Geometry check sheet. Reference: the model listing, model coordinates, mm. Face numbers are marked on the shaded views. A direction names the side the tool comes from. Give positions to 0.01 mm unless a question says otherwise; leave off trailing zeros. Write each loop counter-clockwise with the first axis right and the second up, starting at its lowest first coordinate (ties: lowest second). Pieces come first, ordered by that corner, then holes. Notation, with made-up numbers: (38.25, -8.5) - (68.25, -8.5) arc R14 cw to (68.25, 11.5) - close; hole circle Ø3 at (-16, 7.25). An arc over 180 degrees is marked (long way). Use a Markdown table: item, result.
```python
from build123d import *

# Parameters (mm, degrees)
SKETCH1_R           = 1.5
BOSS_EXTRUDE1_DEPTH = 3


with BuildPart() as part:
    # Sketch1 → Boss-Extrude1 (new body)
    with BuildSketch(Plane.XY):
        with BuildLine():
            Line((84.808392572, 18.957643404), (78, 19.433732591))
            Line((78, 19.433732591), (78, 13))
            ThreePointArc((78, 13), (81.889087297, 11.389087297), (83.5, 7.5))
            Line((83.5, 7.5), (83.5, -7.5))
            ThreePointArc((83.5, -7.5), (81.889087297, -11.389087297), (78, -13))
            Line((78, -13), (78, -19.433732591))
            Line((78, -19.433732591), (84.808392572, -18.957643404))
            ThreePointArc((84.808392572, -18.957643404), (87.805263235, -17.68554728), (89.383648968, -14.838064041))
            Line((89.383648968, -14.838064041), (91.846905706, -0.868240888))
            ThreePointArc((91.846905706, -0.868240888), (91.922866941, 0), (91.846905706, 0.868240888))
            Line((91.846905706, 0.868240888), (89.383648968, 14.838064041))
            ThreePointArc((89.383648968, 14.838064041), (87.805263235, 17.68554728), (84.808392572, 18.957643404))
        make_face()
        with Locations((81, -16)):
            Circle(SKETCH1_R, mode=Mode.SUBTRACT)
        with Locations((81, 16)):
            Circle(SKETCH1_R, mode=Mode.SUBTRACT)
    extrude(amount=BOSS_EXTRUDE1_DEPTH)


solid = part.part
```
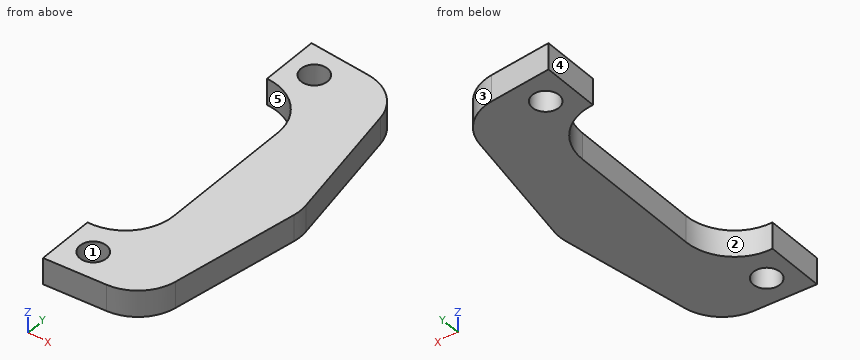
1) Section check B-B on x = 81. Record the boundary of the cut face in (y, z), then the cut area to 3 significant figures.
Working result:
| item | result |
|---|---|
| outline | (-19.22, 0) - (-17.5, 0) - (-17.5, 3) - (-19.22, 3) - close; (-14.5, 0) - (-12.11, 0) - (-12.11, 3) - (-14.5, 3) - close; (12.11, 0) - (14.5, 0) - (14.5, 3) - (12.11, 3) - close; (17.5, 0) - (19.22, 0) - (19.22, 3) - (17.5, 3) - close |
| area | 24.7 mm² |
2) Set-up check for the marked faces 1 and 2: record each of +Z, -Z, +X, -X, +Y, -Y from which the full face is reachable in a straight line by a thin tool's end or side.
Working result:
| item | result |
|---|---|
| face 1 | +Z, -Z |
| face 2 | +Z, -Z, -X |
3) Section check C-C on y = 16. Record the boundary of the cut face in (x, z), then the cut area to 3 significant figures.
Working result:
| item | result |
|---|---|
| outline | (78, 0) - (79.5, 0) - (79.5, 3) - (78, 3) - close; (82.5, 0) - (89.03, 0) - (89.03, 3) - (82.5, 3) - close |
| area | 24.1 mm² |
4) Section check A-A on z = 0.6. Record the boundary of the cut face in (x, y).
Working result:
| item | result |
|---|---|
| outline | (78, -19.43) - (84.81, -18.96) arc R5 ccw to (89.38, -14.84) - (91.85, -0.87) arc R5 ccw to (91.85, 0.87) - (89.38, 14.84) arc R5 ccw to (84.81, 18.96) - (78, 19.43) - (78, 13) arc R5.5 cw to (83.5, 7.5) - (83.5, -7.5) arc R5.5 cw to (78, -13) - close; hole circle Ø3 at (81, -16); hole circle Ø3 at (81, 16) |
5) Depth check by flat-ended pin: P1, Ø3.5, axis at x = 81, y = -16, coming from the +Z side; P2, Ø1.5, axis at y = -3, z = 1, coming from the -X side. Enter the tip coordinate at first touch or a pass-through.
Working result:
| item | result |
|---|---|
| P1 | stops at z = 3 |
| P2 | stops at x = 83.5 |
6) Mould release check, pull along Y, two halves, no side actions. Record for the marked faces 3, 4 and 5: pulls with the +Y half, pulls with the -Y half, needs draft (parallel to the pull), parting line crosses it, or undercut.
Working result:
| item | result |
|---|---|
| face 3 | pulls with the +Y half |
| face 4 | needs draft |
| face 5 | undercut |
7) Material ranges on L1, parallel to Y at x = 81, z = 0.7; L2, parallel to Y at x = 80.25, z = 0.2; L3, parallel to X at y = 17, z = 0.8, recorded low to high. Write a range as from..to.
Working result:
| item | result |
|---|---|
| L1 | y = -19.22..-17.5, -14.5..-12.11, 12.11..14.5, 17.5..19.22 |
| L2 | y = -19.28..-17.3, -14.7..-12.52, 12.52..14.7, 17.3..19.28 |
| L3 | x = 78..79.88, 82.12..88.44 |
8) Section check D-D on y = -14. Record the boundary of the cut face in (x, z), then the cut area to 3 significant figures.
Working result:
| item | result |
|---|---|
| outline | (78, 0) - (89.53, 0) - (89.53, 3) - (78, 3) - close |
| area | 34.6 mm² |
